The model under review builds one solid part; all positions refer to its coordinate system, in mm. Face numbers are marked on the shaded views. Coordinates: 2 decimals unless noted, no trailing zeros. Write each loop counter-clockwise with the first axis right and the second up, starting at its lowest first coordinate (ties: lowest second). Pieces come first, ordered by that corner, then holes. Notation, with made-up numbers: (18.5, -32.75) -> (54.5, -32.75) arc R31 cw to (54.5, 2.25) -> close; hole circle Ø5 at (82.25, 55). An arc over 180 degrees is marked (long way). Write each question's results on one line, items separated by ' | '.
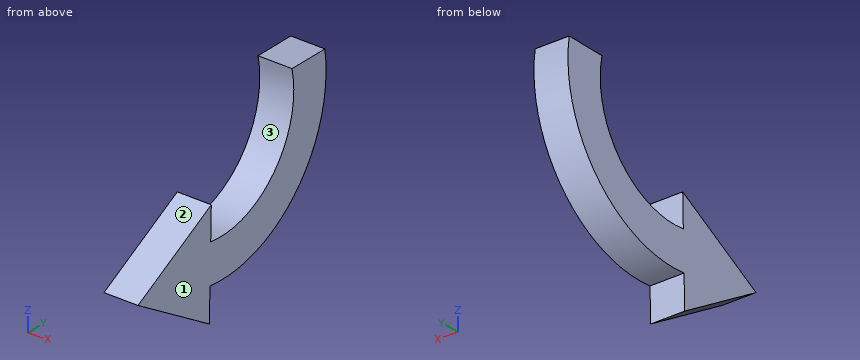
Autodesk Inventor part; units mm, degrees
ref_plane "YZ Plane" through (0, 0, 0) normal (1, 0, 0) x (0, 1, 0)
ref_plane "XZ Plane" through (0, 0, 0) normal (0, 1, 0) x (-1, 0, 0)
ref_plane "XY Plane" through (0, 0, 0) normal (0, 0, 1) x (1, 0, 0)
sketch "Sketch1" plane through (0, 0, 0) normal (1, 0, 0) x (0, 1, 0)
  line L0 (-25.3272, 15.7999) -> (43.5881, 53.4579)
  line L1 (43.5881, 53.4579) -> (41.7432, -25.0535)
  line L2 (41.7432, -25.0535) -> (-25.3272, 15.7999)
  arc A0 (42.3319, 0) -> (150.3078, 111.7735) centre (53.869, 96.8953) ccw
  arc A1 (43.0157, 29.0986) -> (119.4561, 111.7735) centre (52.6501, 96.8661) ccw
  line L3 (119.4561, 111.7735) -> (150.3078, 111.7735)
  point P0 (0, 0)
  point P1 (20.0014, 14.7347)
extrude "Extrusion1" add sketch "Sketch1" along normal blind 25.4
properties part number "Arrow"
Q1. Add section C-C (z = 96.5). Write out the cut boundary in (x, y), plus the area to 3 significant figures.
Solution:
outline: (0, 121.1) -> (25.4, 121.1) -> (25.4, 151.45) -> (0, 151.45) -> close | area: 771 mm²
Q2. Draft analysis for pull direction Z (two halves, no side actions). For the marked faces 1, 2 and 3, state which applies: pulls with the +Z half, pulls with the -Z half, needs draft (parallel to the pull), parting line crosses it, or undercut.
Solution:
face 1: needs draft | face 2: pulls with the +Z half | face 3: undercut
Q3. Clearance check with flat-ended pins moving along their axes: P1, Ø6, axis at x = 16, y = 105, coming from the +Z side; P2, Ø4, axis at x = 13, z = 55.5, coming from the +Y side; P3, Ø3, axis at x = 22, y = 3, coming from the -Z side. State where each tip first meets the part, or that it passes through.
Solution:
P1: z = 56.6 | P2: y = 143.14 | P3: z = -2.37
Q4. Add section A-A (x = 21.75). Write out the cut boundary in (y, z), plus the area to 3 significant figures.
Solution:
outline: (-25.33, 15.8) -> (41.74, -25.05) -> (42.33, 0) arc R97.58 ccw to (150.31, 111.77) -> (119.46, 111.77) arc R68.45 cw to (43.02, 29.1) -> (43.59, 53.46) -> close | area: 7,330 mm²
Q5. For line 1 (Y direction, x = 20, z = 96.5); line 2 (Y direction, x = 15.25, z = 44.5); line 3 (Y direction, x = 15.75, z = 50), list the stretches that pass through material, from the lowest coordinate up. Write a range as from..to.
Solution:
line 1: 121.1..151.45 | line 2: 27.19..43.38, 96.73..136.19 | line 3: 37.26..43.51, 102.54..139.44
Q6. Add section B-B (y = 18.5). Write out the cut boundary in (x, z).
Solution:
outline: (0, -10.9) -> (25.4, -10.9) -> (25.4, 39.75) -> (0, 39.75) -> close
